```python
from build123d import *

# Parameters (mm, degrees)
F1_DEPTH = 45
F3_DEPTH = 45.001
F5_DEPTH = 45.001


with BuildPart() as f1:
    # F0 (on Front) → F1 (new body)
    with BuildSketch(Plane.XZ):
        Polygon((85, 85), (0, 0), (63.63961, 0), (85, 21.36039), align=None)
    extrude(amount=F1_DEPTH)

    # F2 (on face) → F3 (cut, through all)
    with BuildSketch(Plane.XZ.offset(45)):
        Polygon((0, 0), (18.63961, 0), (18.63961, 18.63961), align=None)
    extrude(amount=-F3_DEPTH, mode=Mode.SUBTRACT)

    # F4 (on face) → F5 (cut, through all)
    with BuildSketch(Plane.XZ.offset(45)):
        Polygon((85, 85), (70, 70), (85, 70), align=None)
    extrude(amount=-F5_DEPTH, mode=Mode.SUBTRACT)


solid = f1.part
```
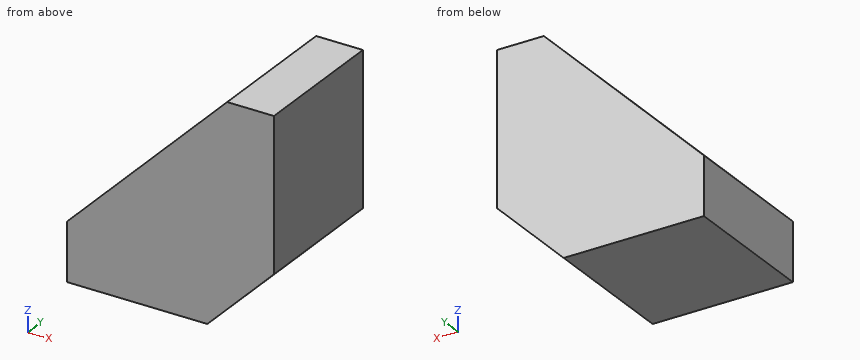
Could you check a few things on this model? Use its own coordinates, in mm. Coordinates: 2 decimals unless noted, no trailing zeros. Loops run counter-clockwise (first coordinate to the right, second up) from the corner with the lowest first, then second, coordinate; pieces in that order, holes last.
1) Please list where these lines run through material, in increasing order: line 1 along X through (y, z) = (-10.5, 63); line 2 along X through (y, z) = (-11, 43); line 3 along Z through (x, y) = (43, -27.5).
Reported:
line 1: x = 63 to 85
line 2: x = 43 to 85
line 3: z = 0 to 43
2) Imagine slicing it at A-A (y = -10.5). List the corners of the cut face in (x, z) for me, and give its area (3 significant figures).
Reported:
outline: (18.64, 0) - (63.64, 0) - (85, 21.36) - (85, 70) - (70, 70) - (18.64, 18.64) - close
area: 3,100 mm2
3) Will these pins go through, and if not, where does the flat tip stop? pin 1 Ø10 at (x, y) = (72.5, -8) entering from -Z; pin 2 Ø12 at (y, z) = (-15.5, 41) entering from -X; pin 3 Ø6 at (y, z) = (-23.5, 48) entering from -X.
Reported:
pin 1: stops at z = 3.86
pin 2: stops at x = 35
pin 3: stops at x = 45
4) Imagine slicing it at B-B (z = 43.5). List the corners of the cut face in (x, y) for me.
Reported:
outline: (43.5, -45) - (85, -45) - (85, 0) - (43.5, 0) - close
5) Imagine slicing it at C-C (x = 53). List the corners of the cut face in (y, z) for me, and give its area (4 significant figures).
Reported:
outline: (-45, 0) - (0, 0) - (0, 53) - (-45, 53) - close
area: 2,385 mm2
